Work out the finished part from the listing and answer in its coordinate system (mm). A direction names the side the tool comes from. Round coordinates to 2 decimals unless told otherwise and drop trailing zeros. Write each loop counter-clockwise with the first axis right and the second up, starting at its lowest first coordinate (ties: lowest second). Pieces come first, ordered by that corner, then holes. Notation, with made-up numbers: M 77,36.5 L 118,36.5 A23 ccw 118,44.5 Z; hole C 45.5,61 d3. An arc over 180 degrees is marked long. One line per item, written item: value. Start each with the question number.
Q1. A tool of negligible diameter and unlimited length cuts with its end or side. For faces 1 (the flat face through (20.469, -0.047, 14.224)), 2 (the flat face through (0, -7.5, 6)), 3 (the flat face through (22.5, 0, 7)), from which of +Z, -Z, +X, -X, +Y, -Y can it reach the whole face along a straight path? Write none if from no direction.
Q2. Consider probe 1 along Y at (x, z) = (19.5, 11.5); probe 2 along X at (y, z) = (6, 12); probe 3 along Z at (x, y) = (9, 8). Determine where each line is inside the solid, lowest interval first.
Q3. The mould has two halves that part along X. Classify faces 4 (the flat face through (-22.5, 0, 8)), 5 (the flat face through (-3, 8, 0)), 6 (the flat face through (20, 0, 7)), 7 (the flat face through (0, 7.5, 6)): released by +X, released by -X, zero draft, split by the parting line, or undercut.
Q4. Find section C-C (y = -4.25). Write down the section's boundary in (x, z), and give its area (3 significant figures).
Q5. Find section A-A (z = 1.75). Write down the section's boundary in (x, y).
Q6. Find section B-B (x = 18.5). Write down the section's boundary in (y, z), and give its area (3 significant figures).
Q7. Find section D-D (z = 13.25). Write down the section's boundary in (x, y).
Q8. Given pin 1 Ø3 at (x, z) = (-4, 9.5) entering from +Y; pin 2 Ø4 at (x, y) = (-6.5, -4.5) entering from +Z (3 decimals), each flat-ended and moving along its own axis, determine where each tip first touches the part or whether it passes through.
from build123d import *

# Parameters (mm, degrees)
F1_DEPTH      = 10
F1_DEPTH_BACK = 10
F2_T          = -2.5


with BuildPart() as f1:
    # F0 (on Front) → F1 (new body, two sides)
    with BuildSketch(Plane.XZ) as f1_sk:
        Polygon((-22.5, 15), (-22.5, 0), (22.5, 0), (22.5, 15), (0, 6.405836), align=None)
    extrude(amount=F1_DEPTH)
    extrude(f1_sk.sketch, amount=-F1_DEPTH_BACK)

    # F2
    f2_openings = [f1.faces().sort_by_distance(p)[0] for p in [
        (0, 0, 0),
        (-11.25, 0, 10.702918),
        (11.25, 0, 10.702918),
    ]]
    offset(amount=F2_T, openings=f2_openings)


solid = f1.part
The answers:
1. face 1: +Z, +Y, -Y
1. face 2: +Z, -Z
1. face 3: +Z, -Z, +X, +Y, -Y
2. probe 1: -10 to -7.5, 7.5 to 10
2. probe 2: -22.5 to -20, 20 to 22.5
2. probe 3: 0 to 9.84
3. face 4: released by -X
3. face 5: zero draft
3. face 6: undercut
3. face 7: undercut
4. outline: M -22.5,0 L -20,0 L -20,14.05 L -22.5,15 Z; M 20,0 L 22.5,0 L 22.5,15 L 20,14.05 Z
4. area: 72.6 mm2
5. outline: M -22.5,-10 L 22.5,-10 L 22.5,10 L -22.5,10 Z; hole M -20,-7.5 L 20,-7.5 L 20,7.5 L -20,7.5 Z
6. outline: M -10,0 L -7.5,0 L -7.5,13.47 L -10,13.47 Z; M 7.5,0 L 10,0 L 10,13.47 L 7.5,13.47 Z
6. area: 67.4 mm2
7. outline: M -22.5,-10 L -17.92,-10 L -17.92,-7.5 L -20,-7.5 L -20,7.5 L -17.92,7.5 L -17.92,10 L -22.5,10 Z; M 17.92,-10 L 22.5,-10 L 22.5,10 L 17.92,10 L 17.92,7.5 L 20,7.5 L 20,-7.5 L 17.92,-7.5 Z
8. pin 1: y = 10
8. pin 2: through
